```python
from build123d import *

# Parameters (mm, degrees)
EXTRUDE_1_DEPTH      = 25
EXTRUDE_2_DEPTH      = 25
EXTRUDE_2_DEPTH_BACK = 20
EXTRUDE_START        = -25
EXTRUDE_3_DEPTH      = 25


with BuildPart() as part:
    # Sketch 2 → Extrude 1 (new body)
    with BuildSketch(Plane(origin=(0, 0, 0), x_dir=(1, 0, 0), z_dir=(0, 1, 0))):
        with BuildLine():
            Line((-50, 0), (-10, 0))
            ThreePointArc((-10, 0), (-9.56304756, 2.923717047), (-8.290375726, 5.591929035))
            Line((-8.290375726, 5.591929035), (-41.451878628, 27.959645174))
            ThreePointArc((-41.451878628, 27.959645174), (-47.815237798, 14.618585236), (-50, 0))
        make_face()
        with BuildLine():
            ThreePointArc((-8.290375726, -5.591929035), (-9.56304756, -2.923717047), (-10, 0))
            Line((-10, 0), (-50, 0))
            ThreePointArc((-50, 0), (-47.815237798, -14.618585236), (-41.451878628, -27.959645174))
            Line((-41.451878628, -27.959645174), (-8.290375726, -5.591929035))
        make_face()
        with BuildLine():
            Line((-10, 0), (-6, 0))
            ThreePointArc((-6, 0), (-5.737828536, 1.754230228), (-4.974225435, 3.355157421))
            Line((-4.974225435, 3.355157421), (-8.290375726, 5.591929035))
            ThreePointArc((-8.290375726, 5.591929035), (-9.56304756, 2.923717047), (-10, 0))
        make_face()
        with BuildLine():
            ThreePointArc((-4.974225435, -3.355157421), (-5.737828536, -1.754230228), (-6, 0))
            Line((-6, 0), (-10, 0))
            ThreePointArc((-10, 0), (-9.56304756, -2.923717047), (-8.290375726, -5.591929035))
            Line((-8.290375726, -5.591929035), (-4.974225435, -3.355157421))
        make_face()
        with BuildLine():
            Line((10, 0), (6, 0))
            ThreePointArc((6, 0), (1.754230228, -5.737828536), (-4.974225435, -3.355157421))
            Line((-4.974225435, -3.355157421), (-8.290375726, -5.591929035))
            ThreePointArc((-8.290375726, -5.591929035), (-4.694715628, -8.829475929), (0, -10))
            ThreePointArc((0, -10), (7.071067812, -7.071067812), (10, 0))
        make_face()
        with BuildLine():
            ThreePointArc((-4.974225435, 3.355157421), (1.754230228, 5.737828536), (6, 0))
            Line((6, 0), (10, 0))
            ThreePointArc((10, 0), (7.071067812, 7.071067812), (0, 10))
            ThreePointArc((0, 10), (-4.694715628, 8.829475929), (-8.290375726, 5.591929035))
            Line((-8.290375726, 5.591929035), (-4.974225435, 3.355157421))
        make_face()
        with BuildLine():
            ThreePointArc((0, 10), (7.071067812, 7.071067812), (10, 0))
            Line((10, 0), (50, 0))
            ThreePointArc((50, 0), (49.74680765, 5.0254481), (48.989794856, 10))
            Line((48.989794856, 10), (0, 10))
        make_face()
        with BuildLine():
            Line((50, 0), (10, 0))
            ThreePointArc((10, 0), (7.071067812, -7.071067812), (0, -10))
            Line((0, -10), (48.989794856, -10))
            ThreePointArc((48.989794856, -10), (49.74680765, -5.0254481), (50, 0))
        make_face()
        with BuildLine():
            Line((53.82, 0), (50, 0))
            ThreePointArc((50, 0), (49.74680765, -5.0254481), (48.989794856, -10))
            Line((48.989794856, -10), (63.82, -10))
            ThreePointArc((63.82, -10), (56.748932188, -7.071067812), (53.82, 0))
        make_face()
        with BuildLine():
            ThreePointArc((48.989794856, 10), (49.74680765, 5.0254481), (50, 0))
            Line((50, 0), (53.82, 0))
            ThreePointArc((53.82, 0), (56.748932188, 7.071067812), (63.82, 10))
            Line((63.82, 10), (48.989794856, 10))
        make_face()
    extrude(amount=EXTRUDE_1_DEPTH)

    # Sketch 2_3 → Extrude 2 (add, two sides: drawn at the far end of the back side and taken through both)
    with BuildSketch(Plane(origin=(0, 0, 0), x_dir=(1, 0, 0), z_dir=(0, 1, 0)).offset(-EXTRUDE_2_DEPTH_BACK)):
        with BuildLine():
            ThreePointArc((63.82, 10), (56.748932188, 7.071067812), (53.82, 0))
            Line((53.82, 0), (63.82, 0))
            Line((63.82, 0), (63.82, 10))
        make_face()
        with BuildLine():
            Line((63.82, 0), (53.82, 0))
            ThreePointArc((53.82, 0), (56.748932188, -7.071067812), (63.82, -10))
            Line((63.82, -10), (63.82, 0))
        make_face()
        with BuildLine():
            Line((63.82, 10), (63.82, 0))
            Line((63.82, 0), (63.82, -10))
            ThreePointArc((63.82, -10), (70.891067812, -7.071067812), (73.82, 0))
            ThreePointArc((73.82, 0), (70.891067812, 7.071067812), (63.82, 10))
        make_face()
    extrude(amount=EXTRUDE_2_DEPTH + EXTRUDE_2_DEPTH_BACK)

    # Sketch 3 → Extrude 3 (add)
    with BuildSketch(Plane(origin=(0, 25, 0), x_dir=(1, 0, 0), z_dir=(0, 1, 0)).offset(EXTRUDE_START)):
        with BuildLine():
            Line((-35.355339059, -35.355339059), (-7.071067812, -7.071067812))
            ThreePointArc((-7.071067812, -7.071067812), (-7.716245834, -6.360782203), (-8.290375726, -5.591929035))
            Line((-8.290375726, -5.591929035), (-41.451878628, -27.959645174))
            ThreePointArc((-41.451878628, -27.959645174), (-38.581229169, -31.803911014), (-35.355339059, -35.355339059))
        make_face()
        with BuildLine():
            ThreePointArc((-8.290375726, 5.591929035), (-7.716245834, 6.360782203), (-7.071067812, 7.071067812))
            Line((-7.071067812, 7.071067812), (-35.355339059, 35.355339059))
            ThreePointArc((-35.355339059, 35.355339059), (-38.581229169, 31.803911014), (-41.451878628, 27.959645174))
            Line((-41.451878628, 27.959645174), (-8.290375726, 5.591929035))
        make_face()
    extrude(amount=EXTRUDE_3_DEPTH)


solid = part.part
```
The model under review builds one solid part; all positions refer to its coordinate system, in mm. A direction names the side the tool comes from. Round coordinates to 2 decimals unless told otherwise and drop trailing zeros. Loops run counter-clockwise (first coordinate to the right, second up) from the corner with the lowest first, then second, coordinate; pieces in that order, holes last. Notation, with made-up numbers: M -22.5,86 L 33.5,86 A32 ccw 33.5,120 Z; hole C 74.5,6 d6. An arc over 180 degrees is marked long. Put each result on its own line as item: value.
Q1. To check wall thickness, follow L1, parallel to Z at x = 46, y = 4.5; L2, parallel to X at y = 2, z = 1.5; L3, parallel to Y at x = 50, z = 6.5. State the ranges of each line that lie inside material, in increasing order.
Result set:
L1: z = -10 to 10
L2: x = -49.98 to -5.81, 5.81 to 73.71
L3: y = 0 to 25
Q2. Consider section A-A, the plane y = 21.5. Give the boundary of the cut face in (x, z), then the cut area to 3 significant figures.
Result set:
outline: M -35.36,-35.36 L -7.07,-7.07 A10 ccw 0,-10 L 63.82,-10 A10 ccw 63.82,10 L 0,10 A10 ccw -7.07,7.07 L -35.36,35.36 A50 ccw Z; hole C 0,0 d12
area: 3,360 mm²
Q3. Mouldability with a two-part tool opening along X and no side actions: class faces 1 (the cylindrical face through (-3.78, 12.32, -9.26)), 2 (the flat face through (64, -20, 0)) as released by +X, released by -X, zero draft, split by the parting line, or undercut.
Result set:
face 1: undercut
face 2: zero draft
Q4. Consider section C-C, the plane x = 56. Give the boundary of the cut face in (y, z), then the cut area to 3 significant figures.
Result set:
outline: M -20,-6.23 L 0,-6.23 L 0,-10 L 25,-10 L 25,10 L 0,10 L 0,6.23 L -20,6.23 Z
area: 749 mm²
Q5. Consider section D-D, the plane z = -14. Give the boundary of the cut face in (x, y).
Result set:
outline: M -48,0 L -14,0 L -14,25 L -48,25 Z
Q6. Consider section B-B, the plane x = 4. Give the boundary of the cut face in (y, z), then the cut area to 3 significant figures.
Result set:
outline: M 0,-10 L 25,-10 L 25,-4.47 L 0,-4.47 Z; M 0,4.47 L 25,4.47 L 25,10 L 0,10 Z
area: 276 mm²
Q7. For pin 1 (10 mm diameter, centred on x = 34.5, y = 2, fed in from -Z); pin 2 (6 mm diameter, centred on x = -32.5, z = -22, fed in from -Y); pin 3 (6 mm diameter, centred on y = 13.5, z = -20.5, fed in from +X), all flat-tipped, find the tip position at first contact; note any pin that passes through.
Result set:
pin 1: stops at z = -10
pin 2: stops at y = 0
pin 3: stops at x = -17.5
Q8. Machinability: for faces 3 (the flat face through (32, 12, -10)), 4 (the flat face through (-3, 25, 7)), 5 (the flat face through (31, 12, 10)), 6 (the cylindrical face through (-3.878, 12.325, 9.218)), which of the approach directions +Z, -Z, +X, -X, +Y, -Y give a long, thin tool a straight path to every point of the face, cutting with its end or side? Answer none if there is none.
Result set:
face 3: -Z, +X, +Y, -Y
face 4: +Z, -Z, +X, -X, +Y
face 5: +Z, +X, +Y, -Y
face 6: +Z, +Y, -Y
